The listing builds one solid part. Answer for the finished solid, in the listing's coordinates (mm). Face numbers are marked on the shaded views. A direction names the side the tool comes from. Coordinates: 2 decimals unless noted, no trailing zeros. Order: outer loops, then holes, each group sorted by start corner. A loop starts at its lowest first (then second) coordinate and runs counter-clockwise, first axis right, second up. Notation, with made-up numbers: (0.5, -15) -> (56.5, -15) arc R18 cw to (56.5, -8) -> close; hole circle Ø9 at (10, 54.5). An arc over 180 degrees is marked (long way). Put each result on its own line as item: value. Start each with the question number.
```python
from build123d import *

# Parameters (mm, degrees)
SKETCH1_W           = 12.2
SKETCH1_H           = 23.1
BOSS_EXTRUDE3_DEPTH = 24.2
SKETCH5_W           = 12.2
SKETCH5_H           = 2.7
BOSS_EXTRUDE4_DEPTH = 4.7
CUT_EXTRUDE4_START  = -20.7
SKETCH6_R           = 1.5
CUT_EXTRUDE4_DEPTH  = 26.2
SKETCH7_R           = 2.75
SKETCH7_R_2         = 6.05
BOSS_EXTRUDE5_DEPTH = 4.5
SKETCH8_R           = 2.5
BOSS_EXTRUDE6_DEPTH = 3


with BuildPart() as part:
    # Sketch1 → Boss-Extrude3 (new body)
    with BuildSketch(Plane(origin=(0, 0, 0), x_dir=(1, 0, 0), z_dir=(0, 1, 0))):
        Rectangle(SKETCH1_W, SKETCH1_H)
    extrude(amount=BOSS_EXTRUDE3_DEPTH)

    # Sketch5 → Boss-Extrude4 (add)
    with BuildSketch(Plane.XY.offset(11.55)):
        with Locations((0, 18.35)):
            Rectangle(SKETCH5_W, SKETCH5_H)
    boss_extrude4 = extrude(amount=BOSS_EXTRUDE4_DEPTH)

    # Sketch6 → Cut-Extrude4 (cut)
    with BuildSketch(Plane(origin=(0, 19.7, 0), x_dir=(1, 0, 0), z_dir=(0, 1, 0)).offset(CUT_EXTRUDE4_START)):
        with Locations((0, -14.25)):
            Circle(SKETCH6_R)
    cut_extrude4 = extrude(amount=CUT_EXTRUDE4_DEPTH, mode=Mode.SUBTRACT)

    # Mirror3: Boss-Extrude4, Cut-Extrude4 across plane
    add(boss_extrude4.mirror(Plane.XY))
    add(cut_extrude4.mirror(Plane.XY), mode=Mode.SUBTRACT)

    # Sketch7 → Boss-Extrude5 (add)
    with BuildSketch(Plane(origin=(0, 24.2, 0), x_dir=(1, 0, 0), z_dir=(0, 1, 0))):
        with Locations((0, -1.2)):
            Circle(SKETCH7_R)
        with Locations((0, 5.5)):
            Circle(SKETCH7_R_2)
    extrude(amount=BOSS_EXTRUDE5_DEPTH)

    # Sketch8 → Boss-Extrude6 (add)
    with BuildSketch(Plane(origin=(0, 28.7, 0), x_dir=(1, 0, 0), z_dir=(0, 1, 0))):
        with Locations((0, 5.5)):
            Circle(SKETCH8_R)
    extrude(amount=BOSS_EXTRUDE6_DEPTH)


solid = part.part
```
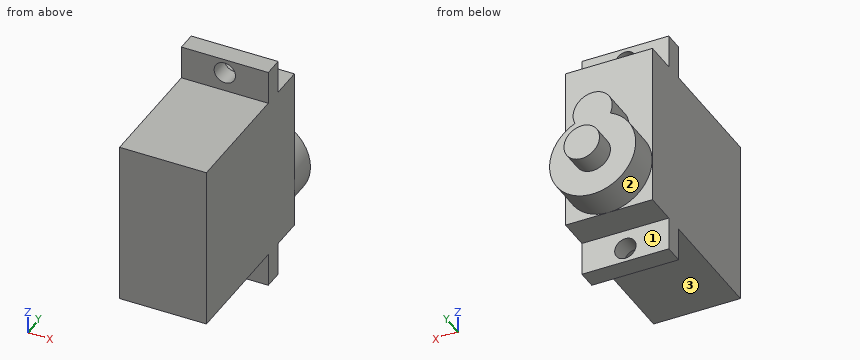
(1) The part is cut by section A-A on z = 14.25. Determine the outline of the cut face in (x, y).
(2) The part is cut by section C-C on x = 5. Determine the outline of the cut face in (y, z), plus the area to 3 significant figures.
(3) Each of these flat-tipped pins is pushed along its axis until it touches: P1, Ø1.4, axis at x = -1, z = 13.5, coming from the +Y side; P2, Ø2, axis at x = -4, z = 5, coming from the +Y side; P3, Ø5, axis at x = 0, y = 26, coming from the -Z side. Where does it stop, or does it pass through?
(4) The part is cut by section D-D on x = -3.25. Determine the outline of the cut face in (y, z).
(5) Find the intervals of material crossed by L1, parallel to Z at x = 0, y = 18.55; L2, parallel to Z at x = 4.25, y = 22; L3, parallel to Y at x = -5.5, z = 9, in increasing order.
(6) A tool of negligible diameter and unlimited length cuts with its end or side. For the marked faces 1, 2 and 3, from which of +Z, -Z, +X, -X, +Y, -Y can it reach the whole face along a straight path? Write none if from no direction.
(7) The part is cut by section B-B on z = -5.5. Determine the outline of the cut face in (x, y).
Worked out:
1. outline: (-6.1, 17) -> (-1.5, 17) -> (-1.5, 19.7) -> (-6.1, 19.7) -> close; (1.5, 17) -> (6.1, 17) -> (6.1, 19.7) -> (1.5, 19.7) -> close
2. outline: (0, -11.55) -> (17, -11.55) -> (17, -16.25) -> (19.7, -16.25) -> (19.7, -11.55) -> (24.2, -11.55) -> (24.2, -8.91) -> (28.7, -8.91) -> (28.7, -2.09) -> (24.2, -2.09) -> (24.2, 11.55) -> (19.7, 11.55) -> (19.7, 16.25) -> (17, 16.25) -> (17, 11.55) -> (0, 11.55) -> close
2. area: 615 mm2
3. P1: y = 19.7
3. P2: y = 24.2
3. P3: z = -11.55
4. outline: (0, -11.55) -> (17, -11.55) -> (17, -16.25) -> (19.7, -16.25) -> (19.7, -11.55) -> (24.2, -11.55) -> (24.2, -10.6) -> (28.7, -10.6) -> (28.7, -0.4) -> (24.2, -0.4) -> (24.2, 11.55) -> (19.7, 11.55) -> (19.7, 16.25) -> (17, 16.25) -> (17, 11.55) -> (0, 11.55) -> close
5. L1: -16.25 to -15.75, -12.75 to 12.75, 15.75 to 16.25
5. L2: -11.55 to 11.55
5. L3: 0 to 24.2
6. face 1: -Z, +X, -X, +Y
6. face 2: +Y
6. face 3: -Z, +X, -X, -Y
7. outline: (-6.1, 0) -> (6.1, 0) -> (6.1, 24.2) -> (6.05, 24.2) -> (6.05, 28.7) -> (2.5, 28.7) -> (2.5, 31.7) -> (-2.5, 31.7) -> (-2.5, 28.7) -> (-6.05, 28.7) -> (-6.05, 24.2) -> (-6.1, 24.2) -> close
